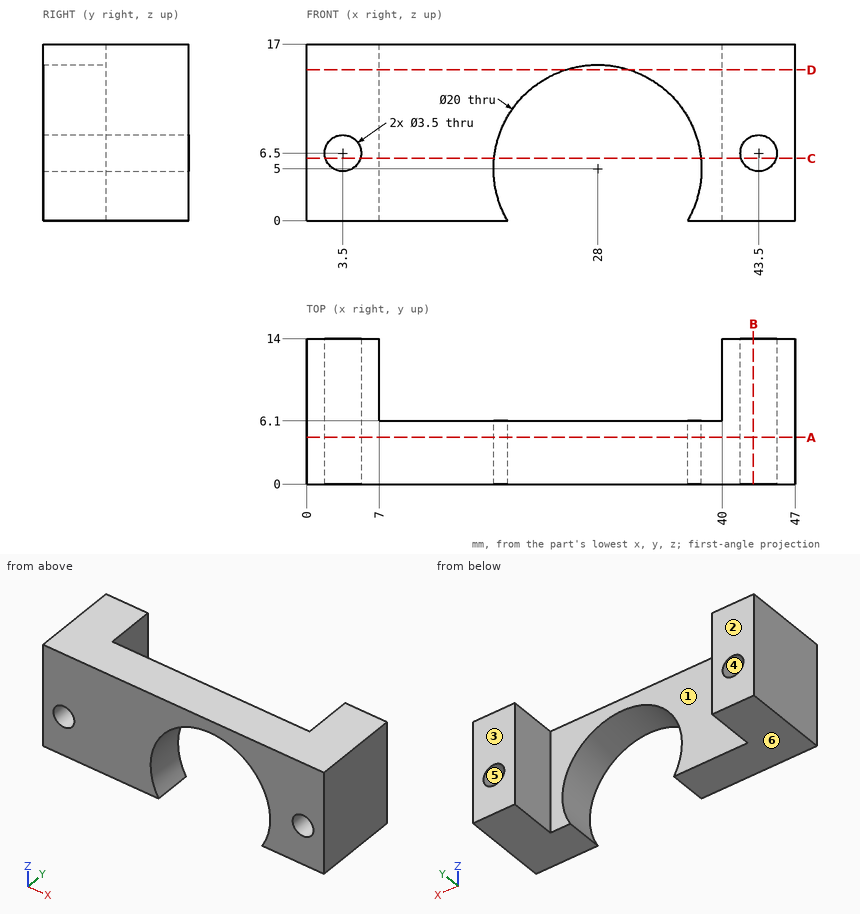
Could you check a few things on this drawing? It's one solid part, dimensions in mm from its lowest x, y, z. A direction names the side the tool comes from. Round coordinates to 2 decimals unless told otherwise and drop trailing zeros. Order: outer loops, then holes, each group sorted by start corner. A loop starts at its lowest first (then second) coordinate and runs counter-clockwise, first axis right, second up.
(1) Imagine slicing it at B-B (x = 43). Write out the boundary of the cut face in (y, z), plus the area to 3 significant figures.
Response values:
outline: (0, 0) - (14, 0) - (14, 4.82) - (0, 4.82) - close; (0, 8.18) - (14, 8.18) - (14, 17) - (0, 17) - close
area: 191 mm2
(2) Imagine slicing it at C-C (z = 6). Write out the boundary of the cut face in (x, y).
Response values:
outline: (0, 0) - (1.82, 0) - (1.82, 14) - (0, 14) - close; (5.18, 0) - (18.05, 0) - (18.05, 6.1) - (7, 6.1) - (7, 14) - (5.18, 14) - close; (37.95, 0) - (41.82, 0) - (41.82, 14) - (40, 14) - (40, 6.1) - (37.95, 6.1) - close; (45.18, 0) - (47, 0) - (47, 14) - (45.18, 14) - close
(3) Please list where these lines run through material, in increasing order: line 1 along Z through (x, y) = (43.5, 4.75); line 2 along X through (y, z) = (9.5, 16); line 3 along Y through (x, z) = (13, 15.5).
Response values:
line 1: z = 0 to 4.75, 8.25 to 17
line 2: x = 0 to 7, 40 to 47
line 3: y = 0 to 6.1
(4) Imagine slicing it at A-A (y = 4.5). Write out the boundary of the cut face in (x, z), plus the area to 3 significant figures.
Response values:
outline: (0, 0) - (19.34, 0) arc R10 cw (long way) to (36.66, 0) - (47, 0) - (47, 17) - (0, 17) - close; hole circle Ø3.5 at (3.5, 6.5); hole circle Ø3.5 at (43.5, 6.5)
area: 527 mm2
(5) Imagine slicing it at D-D (z = 14.5). Write out the boundary of the cut face in (x, y).
Response values:
outline: (0, 0) - (24.88, 0) - (24.88, 6.1) - (7, 6.1) - (7, 14) - (0, 14) - close; (31.12, 0) - (47, 0) - (47, 14) - (40, 14) - (40, 6.1) - (31.12, 6.1) - close
(6) I'm going to push flat-ended pins straight in: pin 1 (4 mm diameter, centred on x = 10, y = 10, fed in from +Z); pin 2 (8 mm diameter, centred on x = 38.5, y = 7, fed in from +Z); pin 3 (5 mm diameter, centred on x = 10, z = 15, fed in from +Y). Where does each tip first touch, or does it pass through?
Response values:
pin 1: passes through
pin 2: stops at z = 17
pin 3: stops at y = 6.1
(7) Which directions (+Z, -Z, +X, -X, +Y, -Y) give clear straight access to the entire face, cutting with the end or side of a thin tool? Please do the marked faces 1 and 2.
Response values:
face 1: +Z, -Z, +Y
face 2: +Z, -Z, +X, -X, +Y
(8) If we mould it in two halves opening along Z, with no side actions, what happens to the marked faces 3, 4, 5 and 6? For each: released by +Z, released by -Z, zero draft, split by the parting line, or undercut.
Response values:
face 3: zero draft
face 4: undercut
face 5: undercut
face 6: released by -Z
